Here's the drawing with two shaded views (mm, measured from the low corner). I have some questions. A direction names the side the tool comes from. Give positions to 0.01 mm unless a question says otherwise; leave off trailing zeros. Order: outer loops, then holes, each group sorted by start corner. A loop starts at its lowest first (then second) coordinate and runs counter-clockwise, first axis right, second up. Notation, with made-up numbers: M 16,20.25 L 46,20.25 A8 ccw 46,30.25 Z; hole C -7.5,15.25 d3. An arc over 180 degrees is marked long. Use a Markdown table: item, result. Add a question column.
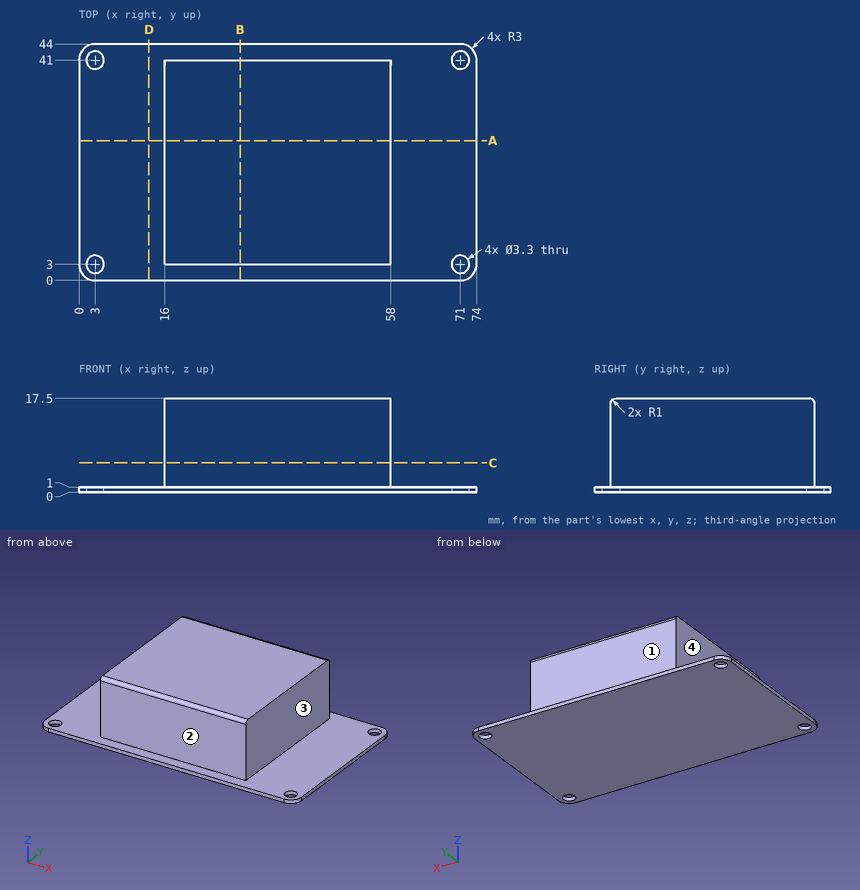
1. If we section it at A-A, the plane y = 26: List the corners of the cut face in (x, z) for me.
2. I need wall thicknesses on L1, parallel to Y at x = 3, z = 0.45; L2, parallel to X at y = 39, z = 9.75; L3, parallel to Y at x = 54.5, z = 9.5. Which ranges of each line are inside material? Lowest first, please. Write a range as [from, to].
3. If we section it at C-C, the plane z = 5.5: List the corners of the cut face in (x, y) for me, then the cut area to 3 significant figures.
4. If we section it at B-B, the plane x = 30: List the corners of the cut face in (y, z) for me, then the cut area to 3 significant figures.
5. If we section it at D-D, the plane x = 13: List the corners of the cut face in (y, z) for me.
6. On a 3-axis mill with a long thin cutter (end or side, diameter ignored), from which of +Z, -Z, +X, -X, +Y, -Y can I reach the whole of each face in a straight line? I mean the marked faces 1, 2, 3 and 4. Say none if no direction works.
7. Will these pins go through, and if not, where does the flat tip stop? pin 1 (2 mm diameter, centred on x = 46, z = 9, fed in from -Y); pin 2 (6 mm diameter, centred on y = 13, z = 8.5, fed in from +X); pin 3 (4 mm diameter, centred on x = 3, y = 41, fed in from +Z); pin 4 (5.5 mm diameter, centred on x = 71, y = 41, fed in from -Z).
Geometry results:
| question | item | result |
|---|---|---|
| 1 | outline | M 0,0 L 74,0 L 74,1 L 58,1 L 58,17.5 L 16,17.5 L 16,1 L 0,1 Z |
| 2 | L1 | y = [0, 1.35], [4.65, 39.35], [42.65, 44] |
| 2 | L2 | x = [16, 58] |
| 2 | L3 | y = [3, 41] |
| 3 | outline | M 16,3 L 58,3 L 58,41 L 16,41 Z |
| 3 | area | 1,600 mm^2 |
| 4 | outline | M 0,0 L 44,0 L 44,1 L 41,1 L 41,16.5 A1 ccw 40,17.5 L 4,17.5 A1 ccw 3,16.5 L 3,1 L 0,1 Z |
| 4 | area | 671 mm^2 |
| 5 | outline | M 0,0 L 44,0 L 44,1 L 0,1 Z |
| 6 | face 1 | +Z, +X, -X, +Y |
| 6 | face 2 | +Z, +X, -X, -Y |
| 6 | face 3 | +Z, +X, +Y, -Y |
| 6 | face 4 | +Z, -X, +Y, -Y |
| 7 | pin 1 | stops at y = 3 |
| 7 | pin 2 | stops at x = 58 |
| 7 | pin 3 | stops at z = 1 |
| 7 | pin 4 | stops at z = 0 |
